Autodesk Inventor part; units mm, degrees
ref_plane "YZ Plane" through (0, 0, 0) normal (1, 0, 0) x (0, 1, 0)
ref_plane "XZ Plane" through (0, 0, 0) normal (0, 1, 0) x (-1, 0, 0)
ref_plane "XY Plane" through (0, 0, 0) normal (0, 0, 1) x (1, 0, 0)
sketch "Sketch1" plane through (0, 0, 0) normal (0, 0, 1) x (1, 0, 0)
  line L0 (-53.3723, 20.7143) -> (51.8738, 20.7143)
  line L1 (51.8738, 20.7143) -> (51.8738, -22.3009)
  line L2 (51.8738, -22.3009) -> (-53.3723, -22.3009)
  line L3 (-53.3723, -22.3009) -> (-53.3723, 20.7143)
  point P0 (0, 0)
extrude "Extrusion1" add sketch "Sketch1" along normal blind 6.35
sketch "Sketch2" plane through (0, 0, 0) normal (0, 0, -1) x (-1, 0, 0)
  line L0 (-51.8738, 20.7143) -> (53.3723, 20.7143)
  line L1 (53.3723, 20.7143) -> (53.3723, -22.3009)
  line L2 (53.3723, -22.3009) -> (-51.8738, -22.3009)
  line L3 (-51.8738, -22.3009) -> (-51.8738, 20.7143)
  line L4 (-47.5602, 15.8741) -> (47.7562, 15.8741)
  line L5 (47.7562, 15.8741) -> (47.7562, -15.8759)
  line L6 (47.7562, -15.8759) -> (-47.5602, -15.8759)
  line L7 (-47.5602, -15.8759) -> (-47.5602, 15.8741)
  line L8 (-50.7352, 19.0491) -> (50.9312, 19.0491)
  line L9 (50.9312, 19.0491) -> (50.9312, -19.0509)
  line L10 (50.9312, -19.0509) -> (-50.7352, -19.0509)
  line L11 (-50.7352, -19.0509) -> (-50.7352, 19.0491)
  line L12 (53.3723, -22.3009) -> (53.3723, 20.7143)
  line L13 (-47.5602, -9.4351) -> (-33.4749, -9.4351)
  line L14 (-33.4749, -9.4351) -> (-29.5119, -13.2742)
  line L15 (-29.5119, -13.2742) -> (-8.1285, -13.2742)
  line L16 (-8.1285, -13.2742) -> (-5.4429, -15.8759)
  point P0 (0, 0)
  dimension "d6" = 3.175
  dimension "d7" = 3.175
  dimension "d8" = 31.75
  dimension "d9" = 3.175
  dimension "d10" = 3.175
extrude "Extrusion2" add sketch "Sketch2" along normal blind 12.7 contours L13 L14 L15 L16 L6 L7 | L8 L9 L10 L11
sketch "Sketch4" plane through (0, 0, -12.7) normal (0, 0, -1) x (-1, 0, 0)
  line L0 (47.7562, -15.8759) -> (-5.4429, -15.8759)
  line L1 (27.7708, -15.8759) -> (39.4699, -15.8759)
  line L2 (39.4699, -15.8759) -> (39.4699, -22.2961)
  line L3 (39.4699, -22.2961) -> (27.7708, -22.2961)
  line L4 (27.7708, -22.2961) -> (27.7708, -15.8759)
  line L5 (-11.0473, -12.4096) -> (-8.1285, -12.4096)
  line L6 (-8.1285, -12.4096) -> (-8.1285, -20.4181)
  line L7 (-8.1285, -20.4181) -> (-11.0473, -20.4181)
  line L8 (-11.0473, -20.4181) -> (-11.0473, -12.4096)
  point P0 (-47.5602, -15.8759)
  point P1 (0, 0)
extrude "Extrusion4" cut sketch "Sketch4" against normal blind 3.175
properties part number "NoiseSourceWell"
The listing builds one solid part. Answer for the finished solid, in the listing's coordinates (mm). A direction names the side the tool comes from. Coordinates: 2 decimals unless noted, no trailing zeros. Loops run counter-clockwise (first coordinate to the right, second up) from the corner with the lowest first, then second, coordinate; pieces in that order, holes last. Notation, with made-up numbers: (85.5, 77) -> (136.5, 77) arc R16 ccw to (136.5, 85) -> close; hole circle Ø3 at (-28.75, 38). An arc over 180 degrees is marked (long way). Write item = value, one per line. Start each with the question number.
1) Given pin 1 Ø2.5 at (y, z) = (-16, -11.5) entering from -X; pin 2 Ø1 at (y, z) = (-18, -10.5) entering from +X; pin 3 Ø6 at (x, z) = (22.5, -9) entering from -Y, each flat-ended and moving along its own axis, determine where each tip first touches the part or whether it passes through.
2) A tool of negligible diameter and unlimited length cuts with its end or side. For faces 1 (the face through (-50.931, 0, -6)), 2 (the face through (-27.771, -17, -11)), 3 (the face through (-47.756, 0, -6)), from which of +Z, -Z, +X, -X, +Y, -Y can it reach the whole face along a straight path? Write none if from no direction.
3) A cutting plane is placed at C-C (y = 14.5). Give the vertices of the cut face in (x, z).
4) The mould has two halves that part along Y. Classify faces 4 (the face through (0, -22.301, 3)), 5 (the face through (31.52, -11.33, -6.26)), 6 (the face through (-39.47, -17, -11)): released by +Y, released by -Y, zero draft, split by the parting line, or undercut.
5) Straight lines are drawn through the part: line 1 (X direction, y = 7.5, z = -2.75); line 2 (Y direction, x = 39.5, z = -1); line 3 (Y direction, x = -26.5, z = -8). For each, find the intervals that lie inside material, in ascending order. Write a range as from..to.
6) A cutting plane is placed at A-A (z = -5). Give the vertices of the cut face in (x, y).
7) A cutting plane is placed at B-B (x = -31.5). Give the vertices of the cut face in (y, z) (3 decimals), then the cut area to 3 significant figures.
Responses:
q1.pin_1 = -50.93
q1.pin_2 = 50.74
q1.pin_3 = -19.05
q2.face_1 = -Z, -X, +Y, -Y
q2.face_2 = -Z, -Y
q2.face_3 = -Z
q3.outline = (-53.37, 0) -> (-50.93, 0) -> (-50.93, -12.7) -> (-47.76, -12.7) -> (-47.76, 0) -> (47.56, 0) -> (47.56, -12.7) -> (50.74, -12.7) -> (50.74, 0) -> (51.87, 0) -> (51.87, 6.35) -> (-53.37, 6.35) -> close
q4.face_4 = released by -Y
q4.face_5 = undercut
q4.face_6 = zero draft
q5.line_1 = -50.93..-47.76, 47.56..50.74
q5.line_2 = -19.05..-9.44, 15.87..19.05
q5.line_3 = -19.05..-15.88, 15.87..19.05
q6.outline = (-50.93, -19.05) -> (50.74, -19.05) -> (50.74, 19.05) -> (-50.93, 19.05) -> close; hole (-47.76, -15.88) -> (5.44, -15.88) -> (8.13, -13.27) -> (29.51, -13.27) -> (33.47, -9.44) -> (47.56, -9.44) -> (47.56, 15.87) -> (-47.76, 15.87) -> close
q7.outline = (-22.301, 0) -> (-19.051, 0) -> (-19.051, -9.525) -> (-15.876, -9.525) -> (-15.876, 0) -> (15.874, 0) -> (15.874, -12.7) -> (19.049, -12.7) -> (19.049, 0) -> (20.714, 0) -> (20.714, 6.35) -> (-22.301, 6.35) -> close
q7.area = 344 mm²
